Job drawing, mm, ordinate dimensions from the low corner. One solid piece. Round coordinates to 2 decimals unless told otherwise and drop trailing zeros. Loops run counter-clockwise (first coordinate to the right, second up) from the corner with the lowest first, then second, coordinate; pieces in that order, holes last.
1) Band-saw the part on D-D, the plane x = 100. Write the cut outline in (y, z), then the cut area to 3 significant figures.
2) Probe line 1 (X direction, y = 2.4, z = 108.5); line 2 (Z direction, x = 14.5, y = 1.45); line 3 (X direction, y = 0.2, z = 69) (1 decimal). List the from-to ranges inside material, lowest first.
3) Band-saw the part on A-A, the plane y = 1.85. Write the cut outline in (x, z) (1 decimal).
4) Drop a flat-ended pin along its axis: P1, Ø1, axis at x = 77, y = 2.5, coming from the +Z side. Give the stop position or say it passes through.
5) Band-saw the part on B-B, the plane x = 83.5. Write the cut outline in (y, z) (1 decimal), then the cut area to 3 significant figures.
6) Band-saw the part on C-C, the plane z = 183. Write the cut outline in (x, y).
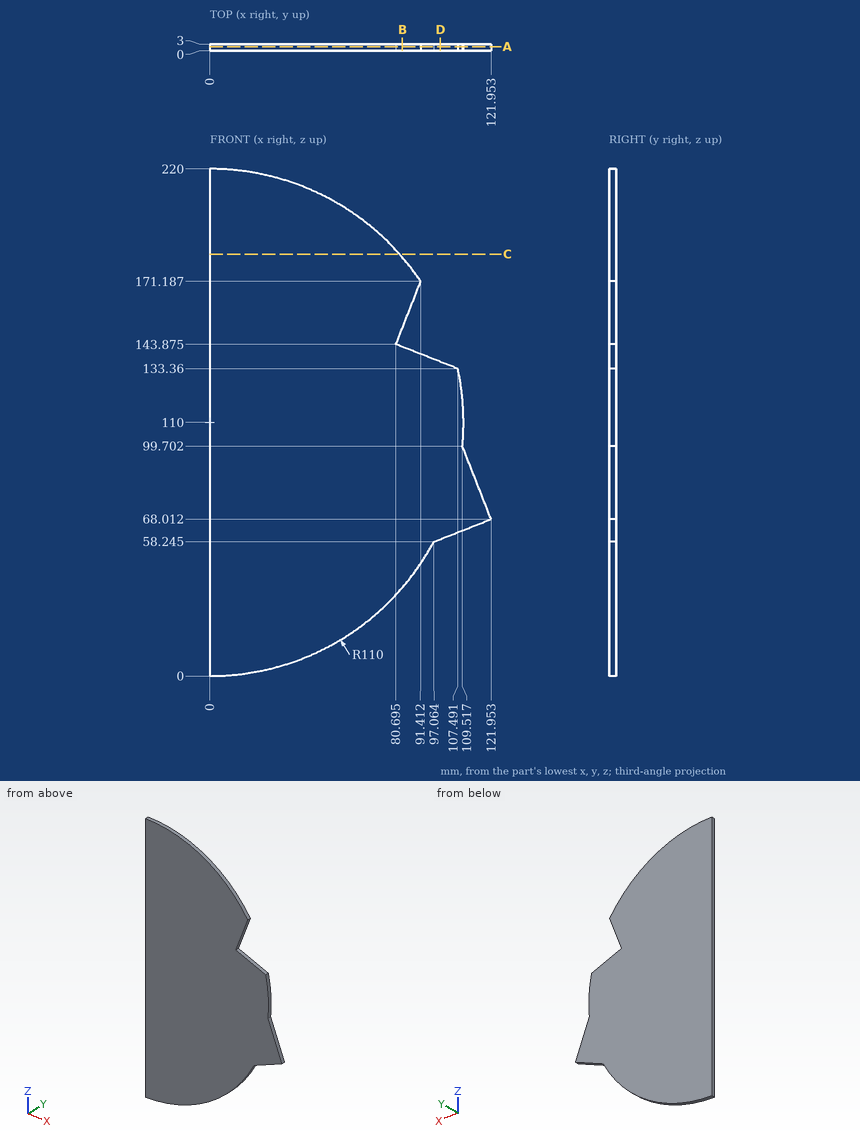
Reported:
1. outline: (0, 59.4) - (3, 59.4) - (3, 136.3) - (0, 136.3) - close
1. area: 231 mm2
2. line 1: x = 0 to 109.99
2. line 2: z = 0.96 to 219.04
2. line 3: x = 0 to 121.6
3. outline: (0, 0) arc R110 ccw to (97.1, 58.2) - (122, 68) - (109.5, 99.7) arc R110 ccw to (107.5, 133.4) - (80.7, 143.9) - (91.4, 171.2) arc R110 ccw to (0, 220) - close
4. P1: stops at z = 189.04
5. outline: (0, 38.4) - (3, 38.4) - (3, 142.8) - (0, 142.8) - close; (0, 151) - (3, 151) - (3, 181.6) - (0, 181.6) - close
5. area: 405 mm2
6. outline: (0, 0) - (82.29, 0) - (82.29, 3) - (0, 3) - close
